Geometry check sheet. Reference: the model listing, model coordinates, mm. Face numbers are marked on the shaded views. A direction names the side the tool comes from. Coordinates: 2 decimals unless noted, no trailing zeros. Order: outer loops, then holes, each group sorted by start corner. A loop starts at its lowest first (then second) coordinate and runs counter-clockwise, first axis right, second up. Notation, with made-up numbers: M 13.25,75.25 L 20.25,75.25 A10 ccw 20.25,93.25 Z; hole C 45.5,-8 d9. An arc over 180 degrees is marked long. Use CSV: the item, a comma, the result in double quotes. Start each with the question number.
```python
from build123d import *

# Parameters (mm, degrees)
SKETCH1_R               = 17.5
BOSS_EXTRUDE1_DEPTH     = 2.5
BOSS_EXTRUDE2_DEPTH     = 8
CUT_EXTRUDE1_DEPTH      = 27.009613607
CUT_EXTRUDE1_DEPTH_BACK = 27.009613607
SKETCH3_R               = 5.5
CUT_EXTRUDE4_START      = -3.5
CUT_EXTRUDE4_DEPTH      = 3.5
SKETCH5_R               = 13
SKETCH5_R_2             = 8
CUT_EXTRUDE5_DEPTH      = 2.2


with BuildPart() as part:
    # Sketch1 → Boss-Extrude1 (new, symmetric)
    with BuildSketch(Plane.XY):
        Circle(SKETCH1_R)
    extrude(amount=BOSS_EXTRUDE1_DEPTH, both=True)

    # Sketch2 → Boss-Extrude2 (add)
    with BuildSketch(Plane.XY.offset(2.5)):
        with BuildLine():
            Line((7.875, 13.63990011), (4.125, 7.144709581))
            ThreePointArc((4.125, 7.144709581), (0, 8.25), (-4.125, 7.144709581))
            Line((-4.125, 7.144709581), (-7.875, 13.63990011))
            ThreePointArc((-7.875, 13.63990011), (0, 15.75), (7.875, 13.63990011))
        make_face()
    extrude(amount=BOSS_EXTRUDE2_DEPTH)

    # Sketch3 → Cut-Extrude1 (cut, two sides: drawn at the far end of the back side and taken through both)
    with BuildSketch(Plane.XY.offset(2.5).offset(-CUT_EXTRUDE1_DEPTH_BACK)):
        Circle(SKETCH3_R)
    extrude(amount=CUT_EXTRUDE1_DEPTH + CUT_EXTRUDE1_DEPTH_BACK, mode=Mode.SUBTRACT)

    # Sketch4 → Cut-Extrude4 (cut)
    with BuildSketch(Plane(origin=(0, 0, -2.5), x_dir=(-1, 0, 0), z_dir=(0, 0, -1)).offset(CUT_EXTRUDE4_START)):
        with BuildLine():
            Line((-3.25, 7.03562364), (-3.25, 4.437059837))
            ThreePointArc((-3.25, 4.437059837), (0, 5.5), (3.25, 4.437059837))
            Line((3.25, 4.437059837), (3.25, 7.03562364))
            ThreePointArc((3.25, 7.03562364), (0, 7.75), (-3.25, 7.03562364))
        make_face()
        with BuildLine():
            Line((3.25, -4.437059837), (3.25, -7.03562364))
            ThreePointArc((3.25, -7.03562364), (0, -7.75), (-3.25, -7.03562364))
            Line((-3.25, -7.03562364), (-3.25, -4.437059837))
            ThreePointArc((-3.25, -4.437059837), (0, -5.5), (3.25, -4.437059837))
        make_face()
        with BuildLine():
            Line((-4.437059837, 3.25), (-7.03562364, 3.25))
            ThreePointArc((-7.03562364, 3.25), (-7.75, 0), (-7.03562364, -3.25))
            Line((-7.03562364, -3.25), (-4.437059837, -3.25))
            ThreePointArc((-4.437059837, -3.25), (-5.5, 0), (-4.437059837, 3.25))
        make_face()
        with BuildLine():
            Line((7.03562364, -3.25), (4.437059837, -3.25))
            ThreePointArc((4.437059837, -3.25), (5.5, 0), (4.437059837, 3.25))
            Line((4.437059837, 3.25), (7.03562364, 3.25))
            ThreePointArc((7.03562364, 3.25), (7.75, 0), (7.03562364, -3.25))
        make_face()
    extrude(amount=CUT_EXTRUDE4_DEPTH, mode=Mode.SUBTRACT)

    # Sketch5 → Cut-Extrude5 (cut)
    with BuildSketch(Plane(origin=(0, 0, -2.5), x_dir=(-1, 0, 0), z_dir=(0, 0, -1))):
        Circle(SKETCH5_R)
        Circle(SKETCH5_R_2, mode=Mode.SUBTRACT)
    extrude(amount=-CUT_EXTRUDE5_DEPTH, mode=Mode.SUBTRACT)


solid = part.part
```
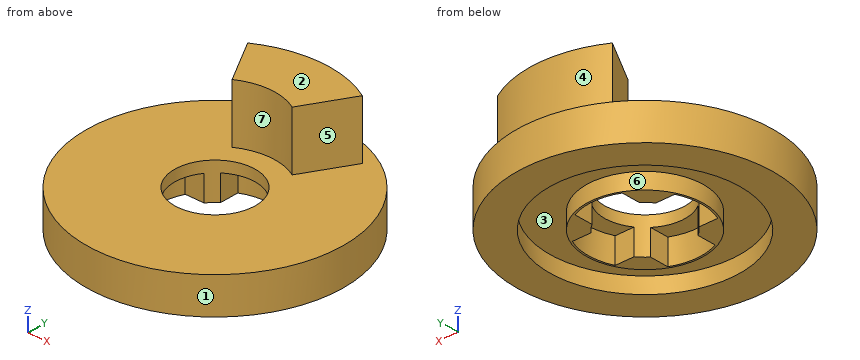
1) Gauge pin test, flat ends, axial feed: P1, Ø6.5, axis at x = 0, y = 0, coming from the +Z side; P2, Ø1, axis at x = -6.5, y = 0.5, coming from the -Z side; P3, Ø3, axis at x = 5, y = -10.5, coming from the +Z side; P4, Ø1.3, axis at x = -6, z = -1.5, coming from the -Y side. Record the tip position at first contact, or that the pin passes through.
2) Section check D-D on y = -12. Record the boundary of the cut face in (x, z).
3) Set-up check for the marked faces 5, 6 and 7: record each of +Z, -Z, +X, -X, +Y, -Y from which the full face is reachable in a straight line by a thin tool's end or side.
4) Section check A-A on x = 0. Record the boundary of the cut face in (y, z).
5) Section check C-C on z = 0.5. Record the boundary of the cut face in (x, y), then the cut area to 3 significant figures.
6) Draft check along Y on the marked faces 1, 2, 3 and 4. Enter one of: +Y half, -Y half, draft (parallel to the pull), parting line (faces both ways), or undercut.
7) Section check B-B on y = 0. Record the boundary of the cut face in (x, z).
8) Material ranges on line 1 along Y through (x, z) = (0, -1.1); line 2 along Y through (x, z) = (0, 1.3); line 3 along Y through (x, z) = (0, 0.4), recorded low to high.
Results are:
1,P1,"passes through"
1,P2,"stops at z = 1"
1,P3,"stops at z = 2.5"
1,P4,"stops at y = -16.66"
2,outline,"M -12.74,-2.5 L -5,-2.5 L -5,-0.3 L 5,-0.3 L 5,-2.5 L 12.74,-2.5 L 12.74,2.5 L -12.74,2.5 Z"
3,face 5,"+Z, +X, -Y"
3,face 6,"-Z"
3,face 7,"+Z, -Y"
4,outline,"M -17.5,-2.5 L -13,-2.5 L -13,-0.3 L -8,-0.3 L -8,-2.5 L -7.75,-2.5 L -7.75,1 L -5.5,1 L -5.5,2.5 L -17.5,2.5 Z; M 5.5,1 L 7.75,1 L 7.75,-2.5 L 8,-2.5 L 8,-0.3 L 13,-0.3 L 13,-2.5 L 17.5,-2.5 L 17.5,2.5 L 15.75,2.5 L 15.75,10.5 L 8.25,10.5 L 8.25,2.5 L 5.5,2.5 Z"
5,outline,"C 0,0 d35; hole M -7.04,-3.25 L -4.44,-3.25 A5.5 ccw -3.25,-4.44 L -3.25,-7.04 A7.75 ccw 3.25,-7.04 L 3.25,-4.44 A5.5 ccw 4.44,-3.25 L 7.04,-3.25 A7.75 ccw 7.04,3.25 L 4.44,3.25 A5.5 ccw 3.25,4.44 L 3.25,7.04 A7.75 ccw -3.25,7.04 L -3.25,4.44 A5.5 ccw -4.44,3.25 L -7.04,3.25 A7.75 ccw Z"
5,area,"806 mm²"
6,face 1,"parting line"
6,face 2,"draft"
6,face 3,"undercut"
6,face 4,"+Y half"
7,outline,"M -17.5,-2.5 L -13,-2.5 L -13,-0.3 L -8,-0.3 L -8,-2.5 L -7.75,-2.5 L -7.75,1 L -5.5,1 L -5.5,2.5 L -17.5,2.5 Z; M 5.5,1 L 7.75,1 L 7.75,-2.5 L 8,-2.5 L 8,-0.3 L 13,-0.3 L 13,-2.5 L 17.5,-2.5 L 17.5,2.5 L 5.5,2.5 Z"
8,line 1,"y = -17.5 to -13, -8 to -7.75, 7.75 to 8, 13 to 17.5"
8,line 2,"y = -17.5 to -5.5, 5.5 to 17.5"
8,line 3,"y = -17.5 to -7.75, 7.75 to 17.5"
